```python
from build123d import *

# Parameters (mm, degrees)
F0_W     = 19.1
F0_H     = 0.8
F0_W_2   = 0.8
F0_H_2   = 13.8
F0_W_3   = 2.45
F0_H_3   = 1
F0_H_4   = 2
F0_W_4   = 4.3
F0_H_5   = 3.875
F0_W_5   = 9.2
F0_H_6   = 3.55
F0_H_7   = 1.25
F1_DEPTH = 1
F2_DEPTH = 2
F3_DEPTH = 5
F4_W     = 2
F4_H     = 2
F4_W_2   = 4.4
F5_DEPTH = 1.5
F6_W     = 2
F6_H     = 2
F7_DEPTH = 2


# Not quite as in the source:
# - a feature names something its author has since deleted; it is built from what else it names


with BuildPart() as f1:
    # F0 (on Top) → F1 (new body)
    with BuildSketch(Plane.XY):
        Polygon((-1.9181339439, 9.1929600332), (-1.1181339439, 9.1929600332), (-1.1181339439, 11.3929600332), (1.0818660561, 11.3929600332), (1.0818660561, 12.1929600332), (-1.1181339439, 12.1929600332), (-1.9181339439, 12.1929600332), align=None)
        Polygon((-1.1181339439, 11.3929600332), (-1.1181339439, 9.1929600332), (1.0818660561, 11.3929600332), align=None)
        with Locations((10.6318660561, 11.7929600332)):
            Rectangle(F0_W, F0_H)
        Polygon((1.0818660561, -6.8070399668), (20.1818660561, -6.8070399668), (22.3818660561, -4.6070399668), (22.3818660561, 0.5179600332), (22.3818660561, 9.1929600332), (20.1818660561, 11.3929600332), (1.0818660561, 11.3929600332), (-1.1181339439, 9.1929600332), (-1.1181339439, -4.6070399668), align=None)
        with Locations((-1.5181339439, 2.2929600332)):
            Rectangle(F0_W_2, F0_H_2)
        Polygon((-1.9181339439, -7.6070399668), (1.0818660561, -7.6070399668), (1.0818660561, -6.8070399668), (-1.1181339439, -6.8070399668), (-1.1181339439, -4.6070399668), (-1.9181339439, -4.6070399668), (-1.9181339439, -6.8070399668), align=None)
        Polygon((-1.1181339439, -6.8070399668), (1.0818660561, -6.8070399668), (-1.1181339439, -4.6070399668), align=None)
        with Locations((10.6318660561, -7.2070399668)):
            Rectangle(F0_W, F0_H)
        Polygon((20.1818660561, -7.6070399668), (23.1818660561, -7.6070399668), (23.1818660561, -4.6070399668), (22.3818660561, -4.6070399668), (22.3818660561, -6.8070399668), (20.1818660561, -6.8070399668), align=None)
        Polygon((22.3818660561, -4.6070399668), (20.1818660561, -6.8070399668), (22.3818660561, -6.8070399668), align=None)
        Polygon((22.3818660561, 0.5179600332), (23.1818660561, 0.5179600332), (23.1818660561, 4.0679600332), (23.1818660561, 5.3179600332), (23.1818660561, 9.1929600332), (22.3818660561, 9.1929600332), align=None)
        Polygon((20.1818660561, 11.3929600332), (22.3818660561, 9.1929600332), (22.3818660561, 11.3929600332), align=None)
        Polygon((22.3818660561, 11.3929600332), (22.3818660561, 9.1929600332), (23.1818660561, 9.1929600332), (23.1818660561, 11.1929600332), (23.1818660561, 12.1929600332), (20.1818660561, 12.1929600332), (20.1818660561, 11.3929600332), align=None)
        with Locations((24.4068660561, 11.6929600332)):
            Rectangle(F0_W_3, F0_H_3)
        with Locations((24.4068660561, 10.1929600332)):
            Rectangle(F0_W_3, F0_H_4)
        with Locations((27.7818660561, 10.1929600332)):
            Rectangle(F0_W_4, F0_H_4)
        with Locations((27.7818660561, 11.6929600332)):
            Rectangle(F0_W_4, F0_H_3)
        with Locations((31.1568660561, 7.2554600332)):
            Rectangle(F0_W_3, F0_H_5)
        Polygon((32.3818660561, 9.1929600332), (32.3818660561, 5.3179600332), (33.1818660561, 5.3179600332), (33.1818660561, 12.1929600332), (32.3818660561, 12.1929600332), (32.3818660561, 11.1929600332), align=None)
        with Locations((27.7818660561, 7.2554600332)):
            Rectangle(F0_W_4, F0_H_5)
        with Locations((24.4068660561, 7.2554600332)):
            Rectangle(F0_W_3, F0_H_5)
        Polygon((23.1818660561, 5.3179600332), (23.1818660561, 4.0679600332), (32.3818660561, 4.0679600332), (32.3818660561, 5.3179600332), (29.9318660561, 5.3179600332), (25.6318660561, 5.3179600332), align=None)
        with Locations((27.7818660561, 2.2929600332)):
            Rectangle(F0_W_5, F0_H_6)
        with Locations((27.7818660561, -0.1070399668)):
            Rectangle(F0_W_5, F0_H_7)
        with Locations((32.7818660561, -0.1070399668)):
            Rectangle(F0_W_2, F0_H_7)
        with Locations((32.7818660561, 2.2929600332)):
            Rectangle(F0_W_2, F0_H_6)
        with Locations((32.7818660561, 4.6929600332)):
            Rectangle(F0_W_2, F0_H_7)
        Polygon((-1.9181339439, 17.1929600332), (-1.9181339439, 12.1929600332), (-1.1181339439, 12.1929600332), (-1.1181339439, 16.3929600332), (23.1818660561, 16.3929600332), (25.6318660561, 16.3929600332), (29.9318660561, 16.3929600332), (32.3818660561, 16.3929600332), (32.3818660561, 12.1929600332), (33.1818660561, 12.1929600332), (33.1818660561, 17.1929600332), (29.9318660561, 17.1929600332), (25.6318660561, 17.1929600332), (23.1818660561, 17.1929600332), align=None)
        Polygon((1.0818660561, 12.1929600332), (20.1818660561, 12.1929600332), (23.1818660561, 12.1929600332), (25.6318660561, 12.1929600332), (29.9318660561, 12.1929600332), (32.3818660561, 12.1929600332), (32.3818660561, 16.3929600332), (29.9318660561, 16.3929600332), (25.6318660561, 16.3929600332), (23.1818660561, 16.3929600332), (-1.1181339439, 16.3929600332), (-1.1181339439, 12.1929600332), align=None)
        Polygon((22.3818660561, -4.6070399668), (23.1818660561, -4.6070399668), (23.1818660561, -0.7320399668), (23.1818660561, 0.5179600332), (22.3818660561, 0.5179600332), align=None)
        with Locations((31.1568660561, 10.1929600332)):
            Rectangle(F0_W_3, F0_H_4)
        with Locations((31.1568660561, 11.6929600332)):
            Rectangle(F0_W_3, F0_H_3)
    extrude(amount=-F1_DEPTH)

    # F0 (on Top) → F2 (join)
    with BuildSketch(Plane.XY):
        Polygon((-1.1181339439, -6.8070399668), (1.0818660561, -6.8070399668), (-1.1181339439, -4.6070399668), align=None)
        Polygon((22.3818660561, -4.6070399668), (20.1818660561, -6.8070399668), (22.3818660561, -6.8070399668), align=None)
        Polygon((20.1818660561, 11.3929600332), (22.3818660561, 9.1929600332), (22.3818660561, 11.3929600332), align=None)
        Polygon((-1.1181339439, 11.3929600332), (-1.1181339439, 9.1929600332), (1.0818660561, 11.3929600332), align=None)
    extrude(amount=F2_DEPTH)

    # F0 (on Top) → F3 (join)
    with BuildSketch(Plane.XY):
        Polygon((-1.9181339439, -7.6070399668), (1.0818660561, -7.6070399668), (1.0818660561, -6.8070399668), (-1.1181339439, -6.8070399668), (-1.1181339439, -4.6070399668), (-1.9181339439, -4.6070399668), (-1.9181339439, -6.8070399668), align=None)
        Polygon((-1.9181339439, 9.1929600332), (-1.1181339439, 9.1929600332), (-1.1181339439, 11.3929600332), (1.0818660561, 11.3929600332), (1.0818660561, 12.1929600332), (-1.1181339439, 12.1929600332), (-1.9181339439, 12.1929600332), align=None)
        Polygon((20.1818660561, -7.6070399668), (23.1818660561, -7.6070399668), (23.1818660561, -4.6070399668), (22.3818660561, -4.6070399668), (22.3818660561, -6.8070399668), (20.1818660561, -6.8070399668), align=None)
        Polygon((22.3818660561, 11.3929600332), (22.3818660561, 9.1929600332), (23.1818660561, 9.1929600332), (23.1818660561, 11.1929600332), (23.1818660561, 12.1929600332), (20.1818660561, 12.1929600332), (20.1818660561, 11.3929600332), align=None)
        Polygon((-1.9181339439, 17.1929600332), (-1.9181339439, 12.1929600332), (-1.1181339439, 12.1929600332), (-1.1181339439, 16.3929600332), (23.1818660561, 16.3929600332), (25.6318660561, 16.3929600332), (29.9318660561, 16.3929600332), (32.3818660561, 16.3929600332), (32.3818660561, 12.1929600332), (33.1818660561, 12.1929600332), (33.1818660561, 17.1929600332), (29.9318660561, 17.1929600332), (25.6318660561, 17.1929600332), (23.1818660561, 17.1929600332), align=None)
        Polygon((32.3818660561, 9.1929600332), (32.3818660561, 5.3179600332), (33.1818660561, 5.3179600332), (33.1818660561, 12.1929600332), (32.3818660561, 12.1929600332), (32.3818660561, 11.1929600332), align=None)
        with Locations((32.7818660561, 4.6929600332)):
            Rectangle(F0_W_2, F0_H_7)
        with Locations((32.7818660561, -0.1070399668)):
            Rectangle(F0_W_2, F0_H_7)
        with Locations((27.7818660561, -0.1070399668)):
            Rectangle(F0_W_5, F0_H_7)
        Polygon((22.3818660561, -4.6070399668), (23.1818660561, -4.6070399668), (23.1818660561, -0.7320399668), (23.1818660561, 0.5179600332), (22.3818660561, 0.5179600332), align=None)
        with Locations((27.7818660561, 10.1929600332)):
            Rectangle(F0_W_4, F0_H_4)
        with Locations((24.4068660561, 10.1929600332)):
            Rectangle(F0_W_3, F0_H_4)
        with Locations((31.1568660561, 10.1929600332)):
            Rectangle(F0_W_3, F0_H_4)
        Polygon((23.1818660561, 5.3179600332), (23.1818660561, 4.0679600332), (32.3818660561, 4.0679600332), (32.3818660561, 5.3179600332), (29.9318660561, 5.3179600332), (25.6318660561, 5.3179600332), align=None)
        with Locations((10.6318660561, -7.2070399668)):
            Rectangle(F0_W, F0_H)
    extrude(amount=F3_DEPTH)

    # F4 (on face) → F5 (join)
    with BuildSketch(Plane.XY.offset(5)):
        with Locations((30.9818660561, 10.1929600332)):
            Rectangle(F4_W, F4_H)
        with Locations((24.5818660561, 10.1929600332)):
            Rectangle(F4_W, F4_H)
        with Locations((27.7818660561, 10.1929600332)):
            Rectangle(F4_W_2, F4_H)
    extrude(amount=F5_DEPTH)

    # F6 (on face) → F7 (join)
    with BuildSketch(Plane.XY.offset(6.5)):
        with Locations((24.5818660561, 10.1929600332)):
            Rectangle(F6_W, F6_H)
        with Locations((30.9818660561, 10.1929600332)):
            Rectangle(F6_W, F6_H)
    extrude(amount=F7_DEPTH)


solid = f1.part
```
The model under review builds one solid part; all positions refer to its coordinate system, in mm. A direction names the side the tool comes from. Give positions to 0.01 mm unless a question says otherwise; leave off trailing zeros. Write each loop counter-clockwise with the first axis right and the second up, starting at its lowest first coordinate (ties: lowest second). Pieces come first, ordered by that corner, then holes. Notation, with made-up numbers: (-5.5, 18.25) -> (52.5, 18.25) arc R26 cw to (52.5, 55.25) -> close; hole circle Ø2 at (6, 85). An arc over 180 degrees is marked (long way). Put each result on its own line as item: value.
(1) To check wall thickness, follow probe 1 along Y at (x, z) = (31, 2); probe 2 along X at (y, z) = (11.75, 4); probe 3 along Y at (x, z) = (2, 4.25). State the ranges of each line that lie inside material, in increasing order. Write a range as from..to.
Results are:
probe 1: -0.73..0.52, 4.07..5.32, 9.19..11.19, 16.39..17.19
probe 2: -1.92..1.08, 20.18..23.18, 32.38..33.18
probe 3: -7.61..-6.81, 16.39..17.19
(2) For pin 1 Ø2.5 at (x, z) = (26.5, 3) entering from -Y; pin 2 Ø1 at (y, z) = (7.5, 1.5) entering from -X; pin 3 Ø0.6 at (y, z) = (10.5, 8) entering from +X, all flat-tipped, find the tip position at first contact; note any pin that passes through.
Results are:
pin 1: y = -0.73
pin 2: x = 32.38
pin 3: x = 31.98
(3) We need section B-B, the plane x = 11. Give the boundary of the cut face in (y, z), and give its area (3 significant figures).
Results are:
outline: (-7.61, -1) -> (17.19, -1) -> (17.19, 5) -> (16.39, 5) -> (16.39, 0) -> (-6.81, 0) -> (-6.81, 5) -> (-7.61, 5) -> close
area: 32.8 mm²
(4) We need section C-C, the plane y = 4.5. Give the boundary of the cut face in (x, z).
Results are:
outline: (-1.92, -1) -> (33.18, -1) -> (33.18, 5) -> (23.18, 5) -> (23.18, 0) -> (-1.92, 0) -> close
(5) Tool access review of faces 4 (the flat face through (23, 11, 5)), 5 (the flat face through (-0.5, -6.2, 2)), 6 (the flat face through (28, 0.518, 2)), 7 (the flat face through (29.982, 10, 7)), 8 (the flat face through (16, -7, 5)): name each direction out of +Z, -Z, +X, -X, +Y, -Y from which nothing blocks a thin tool from reaching the whole face with its end or side.
Results are:
face 4: +Z, -X, +Y, -Y
face 5: +Z
face 6: +Z, +X, -X
face 7: +Z, +Y, -Y
face 8: +Z, +X, -X, -Y
(6) The part is to be moulded in two halves that separate along Y. For faces 1 (the flat face through (25.582, 10, 7)), 2 (the flat face through (10, -7.607, 2)), 3 (the flat face through (23.182, 12, 2)), say which applies: pulls with the +Y half, pulls with the -Y half, needs draft (parallel to the pull), parting line crosses it, or undercut.
Results are:
face 1: needs draft
face 2: pulls with the -Y half
face 3: undercut
